```python
from build123d import *

# Parameters (mm, degrees)
BOSS_EXTRUDE1_DEPTH = 150


with BuildPart() as part:
    # Sketch1 → Boss-Extrude1 (new body, symmetric)
    with BuildSketch(Plane(origin=(0, 0, 0), x_dir=(0, 0, -1), z_dir=(1, 0, 0))):
        with BuildLine():
            Line((-5.05, -0.625), (5.05, -0.625))
            Line((5.05, -0.625), (5.05, 0.141657769))
            ThreePointArc((5.05, 0.141657769), (4.942763552, 0.592183285), (4.644053518, 0.946083289))
            ThreePointArc((4.644053518, 0.946083289), (0, 2.475), (-4.644053518, 0.946083289))
            ThreePointArc((-4.644053518, 0.946083289), (-4.942763552, 0.592183285), (-5.05, 0.141657769))
            Line((-5.05, 0.141657769), (-5.05, -0.625))
        make_face()
    extrude(amount=BOSS_EXTRUDE1_DEPTH, both=True)


solid = part.part
```
The model under review builds one solid part; all positions refer to its coordinate system, in mm. Round coordinates to 2 decimals unless told otherwise and drop trailing zeros. Loops run counter-clockwise (first coordinate to the right, second up) from the corner with the lowest first, then second, coordinate; pieces in that order, holes last. Notation, with made-up numbers: (26, 64) -> (54, 64) arc R24 cw to (54, 87) -> close; hole circle Ø1 at (43.25, 28). An arc over 180 degrees is marked (long way). Answer in a Markdown table with one row per item.
1) Wall thickness on line 1 along Z through (x, y) = (37.5, 0.25); line 2 along Y through (x, z) = (54, 0.75) (3 decimals); line 3 along Y through (x, z) = (44, -1.5) (3 decimals): over which ranges is each line inside the solid? List them lowest first.
Taken from the geometry:
| item | result |
|---|---|
| line 1 | z = -5.04 to 5.04 |
| line 2 | y = -0.625 to 2.439 |
| line 3 | y = -0.625 to 2.33 |
2) Consider section A-A, the plane x = -82.5. Write out the cut boundary in (y, z) (3 decimals).
Taken from the geometry:
| item | result |
|---|---|
| outline | (-0.625, -5.05) -> (0.142, -5.05) arc R1 ccw to (0.946, -4.644) arc R7.818 ccw to (0.946, 4.644) arc R1 ccw to (0.142, 5.05) -> (-0.625, 5.05) -> close |
3) For pin 1 Ø1.5 at (x, y) = (-104, 1) entering from +Z, flat-tipped, find the tip position at first contact; note if it passes through.
Taken from the geometry:
| item | result |
|---|---|
| pin 1 | stops at z = 5.04 |
4) Consider section C-C, the plane z = -2.75. Write out the cut boundary in (x, y) (3 decimals).
Taken from the geometry:
| item | result |
|---|---|
| outline | (-150, -0.625) -> (150, -0.625) -> (150, 1.975) -> (-150, 1.975) -> close |
5) Consider section B-B, the plane y = 1.8. Write out the cut boundary in (x, z), plus the area to 3 significant figures.
Taken from the geometry:
| item | result |
|---|---|
| outline | (-150, -3.18) -> (150, -3.18) -> (150, 3.18) -> (-150, 3.18) -> close |
| area | 1,910 mm² |
